```python
from build123d import *

# Parameters (mm, degrees)
BOSS_EXTRUDE1_DEPTH       = 114
SKETCH2_R                 = 31
CUT_EXTRUDE1_DEPTH        = 61
CUT_EXTRUDE2_DEPTH        = 61
SKETCH5_R                 = 32.5
CUT_EXTRUDE3_DEPTH        = 37
CUT_EXTRUDE4_DEPTH        = 17
SKETCH7_R                 = 19
BOSS_EXTRUDE3_DEPTH       = 3
SKETCH8_W                 = 85.5
SKETCH8_H                 = 10
BOSS_EXTRUDE4_DEPTH       = 3
SKETCH9_W                 = 85.5
SKETCH9_H                 = 10
BOSS_EXTRUDE5_DEPTH       = 3
F_3_0MM_DOWEL_HOLE1_D     = 3
F_3_0MM_DOWEL_HOLE1_DEPTH = 5


with BuildPart() as part:
    # Sketch1 → Boss-Extrude1 (new body)
    with BuildSketch(Plane.XY):
        Polygon((-6.5, 3), (-6.5, 0), (0, 0), (0, 77), (-47.5, 77), (-47.5, 16), (-97, 16), (-102, 0), (-92, 0), (-92, 3), align=None)
        Polygon((0, 77), (0, 0), (6.5, 0), (6.5, 3), (92, 3), (92, 0), (102, 0), (97, 16), (47.5, 16), (47.5, 77), align=None)
    extrude(amount=BOSS_EXTRUDE1_DEPTH)

    # Sketch2 → Cut-Extrude1 (cut)
    with BuildSketch(Plane(origin=(0, 77, 0), x_dir=(1, 0, 0), z_dir=(0, 1, 0))):
        with Locations(Location((0, -57, 0), (0, 0, 180))):  # turned: the seam where the file's is
            Circle(SKETCH2_R)
    extrude(amount=-CUT_EXTRUDE1_DEPTH, mode=Mode.SUBTRACT)

    # Sketch3 → Cut-Extrude2 (cut)
    with BuildSketch(Plane(origin=(0, 77, 0), x_dir=(1, 0, 0), z_dir=(0, 1, 0))):
        with BuildLine():
            Line((-47.5, 0), (-47.5, -57))
            ThreePointArc((-47.5, -57), (0, -9.5), (47.5, -57))
            Line((47.5, -57), (47.5, 0))
            Line((47.5, 0), (-47.5, 0))
        make_face()
        with BuildLine():
            ThreePointArc((47.5, -57), (0, -104.5), (-47.5, -57))
            Line((-47.5, -57), (-47.5, -114))
            Line((-47.5, -114), (47.5, -114))
            Line((47.5, -114), (47.5, -57))
        make_face()
    extrude(amount=-CUT_EXTRUDE2_DEPTH, mode=Mode.SUBTRACT)

    # Sketch5 → Cut-Extrude3 (cut)
    with BuildSketch(Plane(origin=(0, 66, 0), x_dir=(1, 0, 0), z_dir=(0, 1, 0))):
        with Locations(Location((0, -57, 0), (0, 0, 180))):  # turned: the seam where the file's is
            Circle(SKETCH5_R)
    extrude(amount=-CUT_EXTRUDE3_DEPTH, mode=Mode.SUBTRACT)

    # Sketch6 → Cut-Extrude4 (cut, through all)
    with BuildSketch(Plane(origin=(0, 16, 0), x_dir=(1, 0, 0), z_dir=(0, 1, 0))):
        with BuildLine():
            Line((-73, -21), (-67, -21))
            ThreePointArc((-67, -21), (-59, -29), (-67, -37))
            Line((-67, -37), (-73, -37))
            ThreePointArc((-73, -37), (-81, -29), (-73, -21))
        make_face()
        with BuildLine():
            Line((67, -21), (73, -21))
            ThreePointArc((73, -21), (81, -29), (73, -37))
            Line((73, -37), (67, -37))
            ThreePointArc((67, -37), (59, -29), (67, -21))
        make_face()
        with BuildLine():
            Line((67, -77), (73, -77))
            ThreePointArc((73, -77), (81, -85), (73, -93))
            Line((73, -93), (67, -93))
            ThreePointArc((67, -93), (59, -85), (67, -77))
        make_face()
        with BuildLine():
            Line((-73, -77), (-67, -77))
            ThreePointArc((-67, -77), (-59, -85), (-67, -93))
            Line((-67, -93), (-73, -93))
            ThreePointArc((-73, -93), (-81, -85), (-73, -77))
        make_face()
    extrude(amount=-CUT_EXTRUDE4_DEPTH, mode=Mode.SUBTRACT)

    # Sketch7 → Boss-Extrude3 (add)
    with BuildSketch(Plane(origin=(0, 16, 0), x_dir=(1, 0, 0), z_dir=(0, 1, 0))):
        with Locations(Location((-70, -29, 0), (0, 0, 180))):  # turned: the seam where the file's is
            Circle(SKETCH7_R)
        with BuildLine():
            Line((-67, -37), (-73, -37))
            ThreePointArc((-73, -37), (-81, -29), (-73, -21))
            Line((-73, -21), (-67, -21))
            ThreePointArc((-67, -21), (-59, -29), (-67, -37))
        make_face(mode=Mode.SUBTRACT)
        with Locations(Location((70, -29, 0), (0, 0, 180))):  # turned: the seam where the file's is
            Circle(SKETCH7_R)
        with BuildLine():
            Line((73, -37), (67, -37))
            ThreePointArc((67, -37), (59, -29), (67, -21))
            Line((67, -21), (73, -21))
            ThreePointArc((73, -21), (81, -29), (73, -37))
        make_face(mode=Mode.SUBTRACT)
        with Locations(Location((70, -85, 0), (0, 0, 180))):  # turned: the seam where the file's is
            Circle(SKETCH7_R)
        with BuildLine():
            Line((73, -93), (67, -93))
            ThreePointArc((67, -93), (59, -85), (67, -77))
            Line((67, -77), (73, -77))
            ThreePointArc((73, -77), (81, -85), (73, -93))
        make_face(mode=Mode.SUBTRACT)
        with Locations(Location((-70, -85, 0), (0, 0, 180))):  # turned: the seam where the file's is
            Circle(SKETCH7_R)
        with BuildLine():
            Line((-67, -93), (-73, -93))
            ThreePointArc((-73, -93), (-81, -85), (-73, -77))
            Line((-73, -77), (-67, -77))
            ThreePointArc((-67, -77), (-59, -85), (-67, -93))
        make_face(mode=Mode.SUBTRACT)
    extrude(amount=BOSS_EXTRUDE3_DEPTH)

    # Sketch8 → Boss-Extrude4 (add)
    with BuildSketch(Plane(origin=(0, 3, 0), x_dir=(-1, 0, 0), z_dir=(0, -1, 0))):
        with Locations((49.25, -5)):
            Rectangle(SKETCH8_W, SKETCH8_H)
        with Locations((49.25, -109)):
            Rectangle(SKETCH8_W, SKETCH8_H)
    extrude(amount=BOSS_EXTRUDE4_DEPTH)

    # Sketch9 → Boss-Extrude5 (add)
    with BuildSketch(Plane(origin=(0, 3, 0), x_dir=(-1, 0, 0), z_dir=(0, -1, 0))):
        with Locations((-49.25, -109)):
            Rectangle(SKETCH9_W, SKETCH9_H)
        with Locations((-49.25, -5)):
            Rectangle(SKETCH9_W, SKETCH9_H)
    extrude(amount=BOSS_EXTRUDE5_DEPTH)

    # Ø3.0mm Dowel Hole1
    with Locations(Plane(origin=(0, 16, 0), x_dir=(1, 0, 0), z_dir=(0, 1, 0))):
        with Locations((-22, -57)):
            Hole(F_3_0MM_DOWEL_HOLE1_D / 2, depth=F_3_0MM_DOWEL_HOLE1_DEPTH)


solid = part.part
```
CAD build for the part. Positions are in the model's coordinates, mm. A direction names the side the tool comes from. Coordinates: 2 decimals unless noted, no trailing zeros. Loops run counter-clockwise (first coordinate to the right, second up) from the corner with the lowest first, then second, coordinate; pieces in that order, holes last. Notation, with made-up numbers: (27, 82.25) - (55, 82.25) arc R20 ccw to (55, 121.25) - close; hole circle Ø7 at (-1.5, 39.25). An arc over 180 degrees is marked (long way). Return JSON: item names as keys, results as strings.
1. Band-saw the part on B-B (z = 15). Give the cut face in (x, y).
Result:
{"outline": "(-102, 0) - (-92, 0) - (-92, 3) - (-6.5, 3) - (-6.5, 0) - (6.5, 0) - (6.5, 3) - (92, 3) - (92, 0) - (102, 0) - (97, 16) - (82.85, 16) - (82.85, 19) - (57.15, 19) - (57.15, 16) - (22.19, 16) - (22.19, 77) - (-22.19, 77) - (-22.19, 16) - (-57.15, 16) - (-57.15, 19) - (-82.85, 19) - (-82.85, 16) - (-97, 16) - close"}
2. Band-saw the part on A-A (x = -70). Give the cut face in (y, z).
Result:
{"outline": "(0, 0) - (16, 0) - (16, 10) - (19, 10) - (19, 21) - (3, 21) - (3, 10) - (0, 10) - close; (0, 104) - (3, 104) - (3, 93) - (19, 93) - (19, 104) - (16, 104) - (16, 114) - (0, 114) - close; (3, 37) - (19, 37) - (19, 48) - (16, 48) - (16, 66) - (19, 66) - (19, 77) - (3, 77) - close"}
3. Band-saw the part on D-D (y = 48). Give the cut face in (x, z), and give its area (3 significant figures).
Result:
{"outline": "circle Ø95 at (0, 57); hole circle Ø65 at (0, 57)", "area": "3,770 mm2"}
4. Drop flat-ended pins along their axis: pin 1 (1.5 mm diameter, centred on y = 26.5, z = 52.5, fed in from +X); pin 2 (2.5 mm diameter, centred on x = -22, z = 57, fed in from +Y); pin 3 (10 mm diameter, centred on x = 18.5, z = 96, fed in from -Y). Give the stop position or say it passes through.
Result:
{"pin 1": "stops at x = 47.35", "pin 2": "stops at y = 11", "pin 3": "stops at y = 3"}
5. Probe L1, parallel to X at y = 17.5, z = 81.5; L2, parallel to Z at x = 0, y = 71.5; L3, parallel to Y at x = 55, z = 50. List the from-to ranges inside material, lowest first. Write a range as from..to.
Result:
{"L1": "x = -88.67..-80.19, -59.81..-51.33, -40.69..-18.99, 18.99..40.69, 51.33..59.81, 80.19..88.67", "L2": "z = 9.5..26, 88..104.5", "L3": "y = 3..16"}
6. Mould opens along Z. For faces 1 (the flat face through (1, 0, 56)), 2 (the cylindrical face through (-54.92, 17.48, 17.44)), 3 (the flat face through (1, 8, 114)) say: released by +Z, released by -Z, zero draft, split by the parting line, or undercut.
Result:
{"face 1": "zero draft", "face 2": "undercut", "face 3": "released by +Z"}
7. Band-saw the part on C-C (y = 8.5). Give the cut face in (x, z).
Result:
{"outline": "(-99.34, 0) - (99.34, 0) - (99.34, 114) - (-99.34, 114) - close; hole (-73, 21) - (-67, 21) arc R8 ccw to (-67, 37) - (-73, 37) arc R8 ccw to start; hole (-73, 77) - (-67, 77) arc R8 ccw to (-67, 93) - (-73, 93) arc R8 ccw to start; hole (67, 21) - (73, 21) arc R8 ccw to (73, 37) - (67, 37) arc R8 ccw to start; hole (67, 77) - (73, 77) arc R8 ccw to (73, 93) - (67, 93) arc R8 ccw to start"}
8. 3-axis set-ups, long thin cutter, end or side, ignore diameter. For faces 4 (the cylindrical face through (22.85, 22.59, 77.95)), 5 (the flat face through (-70, 11, 37)), 6 (the flat face through (70.3, 19, 76.8)): which of +Z, -Z, +X, -X, +Y, -Y reach the whole face in a straight line?
Result:
{"face 4": "+Y", "face 5": "+Y, -Y", "face 6": "+Z, -Z, +X, +Y"}
